Source: CAD feature listing. Evaluate the final solid. Frame: model axes, mm. A direction names the side the tool comes from. Round coordinates to 2 decimals unless told otherwise and drop trailing zeros. Write each loop counter-clockwise with the first axis right and the second up, starting at its lowest first coordinate (ties: lowest second). Pieces come first, ordered by that corner, then holes.
Autodesk Inventor part; units mm, degrees
ref_plane "YZ Plane" through (0, 0, 0) normal (1, 0, 0) x (0, 1, 0)
ref_plane "XZ Plane" through (0, 0, 0) normal (0, 1, 0) x (-1, 0, 0)
ref_plane "XY Plane" through (0, 0, 0) normal (0, 0, 1) x (1, 0, 0)
sketch "Эскиз24" plane through (0, 0, 0) normal (0, 1, 0) x (1, 0, 0)
  line L0 (0, 0) -> (24.5, 0)
  line L1 (24.5, 0) -> (24.5, 17)
  line L2 (24.5, 17) -> (0, 17)
  line L3 (0, 17) -> (0, 0)
  dimension "d124" = 24.5
  dimension "d125" = 17
extrude "Выдавливание17" add sketch "Эскиз24" along normal blind 4.5
sketch "Эскиз25" plane through (0, 4.5, 0) normal (0, 1, 0) x (1, 0, 0)
  line L0 (24.5, 1) -> (7, 1)
  line L1 (7, 1) -> (7, 16)
  line L2 (7, 16) -> (24.5, 16)
  line L3 (24.5, 16) -> (24.5, 1)
  line L4 (24.5, 0) -> (24.5, 17)
  line L5 (0, 17) -> (0, 0)
  point P0 (24.5, 8.5)
  dimension "d128" = 15
  dimension "d129" = 17.5
extrude "Выдавливание18" cut sketch "Эскиз25" against normal blind 3.5
sketch "Эскиз26" plane through (0, 4.5, 0) normal (0, 1, 0) x (1, 0, 0)
  line L0 (7, 1) -> (7, 16)
  line L1 (2, 5.5) -> (7, 5.5)
  line L2 (7, 5.5) -> (7, 11.5)
  line L3 (7, 11.5) -> (2, 11.5)
  line L4 (2, 11.5) -> (2, 5.5)
  line L5 (7, 1) -> (7, 16)
  point P0 (0, 0)
  point P1 (7, 8.5)
  dimension "d133" = 5
  dimension "d134" = 6
extrude "Выдавливание19" cut sketch "Эскиз26" against normal blind 3
fillet "Сопряжение8" radius 3 2 edges at (4.5, 1.5, -11.5) (4.5, 1.5, -5.5)
sketch "Эскиз27" plane through (0, 4.5, 0) normal (0, 1, 0) x (1, 0, 0)
  line L0 (0, 6.5) -> (2, 6.5)
  line L1 (2, 6.5) -> (2, 10.5)
  line L2 (2, 10.5) -> (0, 10.5)
  line L3 (0, 10.5) -> (0, 6.5)
  line L4 (2, 5.5) -> (2, 11.5)
  line L5 (0, 17) -> (0, 0)
  point P0 (2, 8.5)
  dimension "d138" = 4
extrude "Выдавливание20" cut sketch "Эскиз27" against normal blind 2
fillet "Сопряжение9" radius 2 2 edges at (1, 2.5, -10.5) (1, 2.5, -6.5)
sketch "Эскиз28" plane through (0, 4.5, 0) normal (0, 1, 0) x (1, 0, 0)
  line L0 (2, 11.5) -> (7, 11.5)
  line L1 (0, 17) -> (0, 0)
  line L2 (7, 11.5) -> (0, 11.5)
  line L3 (0, 11.5) -> (0, 17)
  line L4 (0, 17) -> (7, 17)
  line L5 (7, 17) -> (7, 11.5)
  line L6 (7, 5.5) -> (2, 5.5)
  line L7 (7, 5.5) -> (0, 5.5)
  line L8 (0, 5.5) -> (0, 0)
  line L9 (0, 0) -> (7, 0)
  line L10 (7, 0) -> (7, 5.5)
  line L11 (24.5, 17) -> (0, 17) construction
  line L12 (0, 17) -> (7, 11.5) construction
  line L13 (0, 0) -> (7, 5.5) construction
  point P0 (3.5, 14.25)
  point P1 (3.5, 2.75)
hole "Отверстие6" at (3.5, 4.5, -14.25) at (3.5, 4.5, -2.75) direction (0, -1, 0) diameter 2 depth 4.5
sketch "Эскиз21" plane through (20, 0, 0.1742) normal (1, 0, 0) x (0, 0, -1)
  line L0 (0.1742, 0) -> (-5.0258, 0)
  line L1 (0.1742, 0) -> (0.1742, 25)
  line L2 (-5.0258, 0) -> (-8.7758, -17.85)
  line L3 (0.1742, 0) -> (-3.5758, -17.85)
  line L4 (-8.7758, -17.85) -> (-3.5758, -17.85)
  dimension "d103" = 17.85
  dimension "d104" = 8.95
sketch "Эскиз22" plane through (20, -17.85, 3.75) normal (0, -1, 0) x (1, 0, 0)
  line L0 (0, 0) -> (-9.1, 0)
  line L1 (-9.1, 0) -> (-9.1, 17.3)
  line L2 (-9.1, 17.3) -> (0, 17.3)
  line L3 (0, 17.3) -> (0, 0)
  line L4 (0, 5.2) -> (-9.1, 5.2)
  line L5 (0, 0) -> (-9.1, 0)
  line L6 (0, 5.2) -> (0, 0)
  line L7 (0, 0) -> (-9.1, 0)
  line L8 (-9.1, 0) -> (-9.1, 5.2)
  line L9 (0, 5.2) -> (-9.1, 5.2)
  point P0 (-20, -3.75)
  point P1 (0, -7.9181)
  point P2 (-9.1, -7.9181)
  point P3 (-9.1, 0)
  point P4 (-9.1, -7.9181)
  point P5 (0, -7.9181)
  point P6 (0, 0)
  point P7 (0, 4.1819)
  point P8 (-9.1, 4.1819)
  dimension "d122" = 12.1
sketch "Эскиз23" plane through (40.15, -13.85, 3.75) normal (0, 1, 0) x (1, 0, 0)
  line L0 (-9.1, -17.3) -> (0, -17.3)
  line L1 (-4.55, -17.3) -> (-4.55, -12.6)
  point P0 (-40.15, 3.75)
  dimension "d118" = 4.7
properties part number "Крепление USB"
Q1. Section query D-D, the plane x = 13.75. Output: boundary loops of the cut face in (y, z).
Q2. Line query: line 1 (Z direction, x = 3.5, y = 1.05); line 2 (Z direction, x = 16.75, y = 3.05); line 3 (X direction, y = 1.65, z = -2.75). Output: solid intervals per line, ascending.
Q3. Mould query, pull axis X, two halves, no side actions, for faces 1 (the face through (3.2, 2.218, -13.296)), 2 (the face through (0, 2, -9)), 3 (the face through (4.46, 2.4, -10.64)). Classes: pulls with the +X half, pulls with the -X half, needs draft (parallel to the pull), parting line crosses it, or undercut.
Q4. Set-up query: faces 4 (the face through (24.5, 0.7, -8.5)), 5 (the face through (16, 3, -16)), 6 (the face through (0.99, 3.1, -9.93)). Return all of +Z, -Z, +X, -X, +Y, -Y with unobstructed straight access to the full face (end or side cutting, diameter ignored); none if empty.
Q5. Section query B-B, the plane x = 3.5. Give the number of separate pieces and of enclosed holes in the cut face, and give its area (3 significant figures).
Q6. Section query A-A, the plane z = -2.75. Output: boundary loops of the cut face in (x, y).
Q7. Section query C-C, the plane y = 4.1. Output: boundary loops of the cut face in (x, z).
Q8. Pin query (flat end, axial travel): P1, Ø1.5, axis at y = 3, z = -8.5, coming from the +X side; P2, Ø1.8, axis at x = 3.5, z = -2.75, coming from the +Y side; P3, Ø4.5, axis at x = 13, z = -9.5, coming from the +Y side. Return the tip coordinate at first contact, or that it passes through.
Filled in:
1. outline: (0, -17) - (4.5, -17) - (4.5, -16) - (1, -16) - (1, -1) - (4.5, -1) - (4.5, 0) - (0, 0) - close
2. line 1: z = -17 to -15.25, -13.25 to -3.75, -1.75 to 0
2. line 2: z = -17 to -16, -1 to 0
2. line 3: x = 0 to 2.5, 4.5 to 7
3. face 1: undercut
3. face 2: pulls with the -X half
3. face 3: needs draft
4. face 4: +Z, -Z, +X, +Y, -Y
4. face 5: +X, +Y
4. face 6: +X, -X, +Y
5. separate pieces: 3
5. enclosed holes: 0
5. area: 44.4 mm2
6. outline: (0, 0) - (2.5, 0) - (2.5, 4.5) - (0, 4.5) - close; (4.5, 0) - (24.5, 0) - (24.5, 1) - (7, 1) - (7, 4.5) - (4.5, 4.5) - close
7. outline: (0, -17) - (24.5, -17) - (24.5, -16) - (7, -16) - (7, -11.47) - (2, -11.47) - (2, -10.46) - (0, -10.46) - close; (0, -6.54) - (2, -6.54) - (2, -5.53) - (7, -5.53) - (7, -1) - (24.5, -1) - (24.5, 0) - (0, 0) - close; hole circle Ø2 at (3.5, -14.25); hole circle Ø2 at (3.5, -2.75)
8. P1: stops at x = 2
8. P2: passes through
8. P3: stops at y = 1
